Job drawing, mm, ordinate dimensions from the low corner. One solid piece. Round coordinates to 2 decimals unless told otherwise and drop trailing zeros. Write each loop counter-clockwise with the first axis right and the second up, starting at its lowest first coordinate (ties: lowest second). Pieces come first, ordered by that corner, then holes. Notation, with made-up numbers: (34.25, 54) -> (92.25, 54) arc R7 ccw to (92.25, 64) -> close; hole circle Ø9 at (-36, 33.25). An arc over 180 degrees is marked (long way). Use CSV: the item, a comma, the result in double quotes. Start each with the question number.
(1) Probe line 1 (X direction, y = 11, z = 8.75) (3 decimals); line 2 (Z direction, x = 13.25, y = 12.75). List the from-to ranges inside material, lowest first. Write a range as [from, to].
(2) Drop a flat-ended pin along its axis: pin 1 (2 mm diameter, centred on x = 11.5, y = 11.5, fed in from +Z). Give the stop position or say it passes through.
(3) Saw through at A-A (y = 11). Give the cut face in (x, z) (3 decimals).
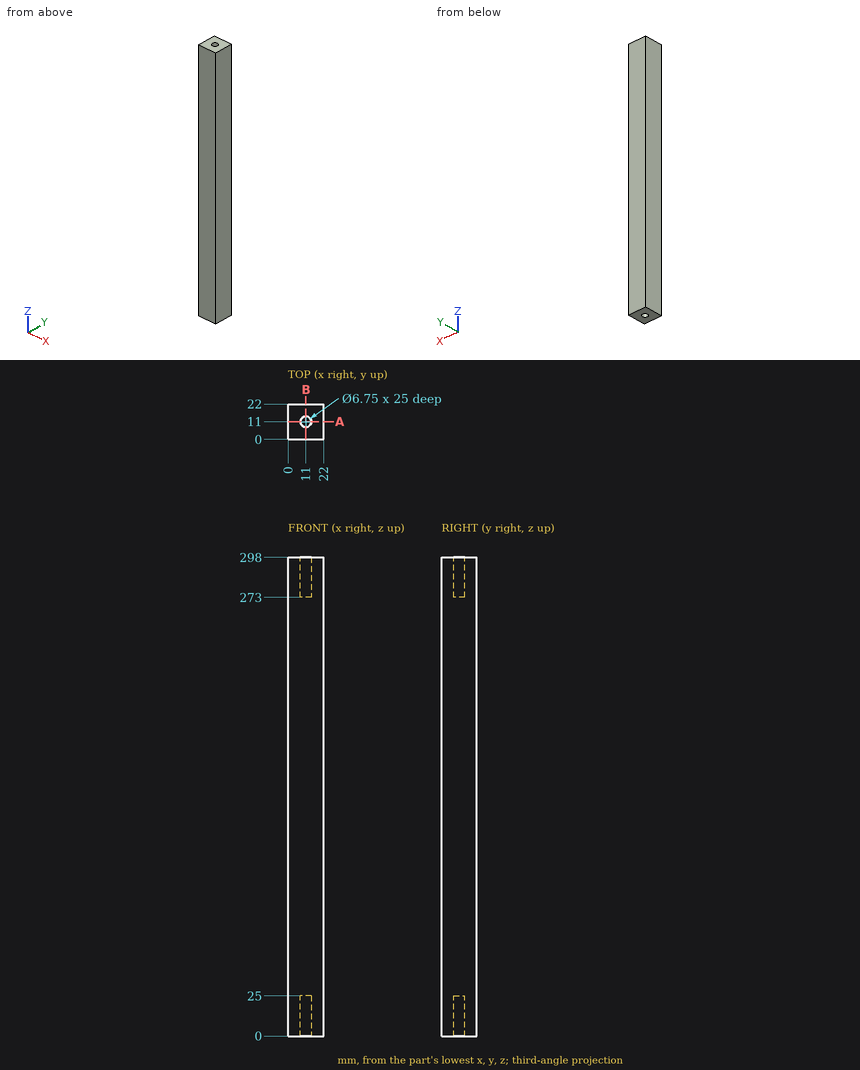
Answers:
1,line 1,"x = [0, 7.625], [14.375, 22]"
1,line 2,"z = [25, 273]"
2,pin 1,"stops at z = 273"
3,outline,"(0, 0) -> (7.625, 0) -> (7.625, 25) -> (14.375, 25) -> (14.375, 0) -> (22, 0) -> (22, 298) -> (14.375, 298) -> (14.375, 273) -> (7.625, 273) -> (7.625, 298) -> (0, 298) -> close"
